```python
from build123d import *

# Parameters (mm, degrees)
F4_W      = 5.05
F4_H      = 5.35
F9_R      = 3
F10_DEPTH = 11.671
F11_R     = 0.5
F12_SIZE  = 0.2


with BuildPart() as f6:
    # F6: sweep along a path in F1
    with BuildLine(Plane.XZ) as f6_path:
        Line((0, 0), (0, 1.2))
        Line((0, 1.2), (0, 3.4))
        Line((0, 3.4), (0, 4.67))
        Line((0, 4.67), (0, 11.67))
    # F5 (on Top) → F6 (sweep)
    with BuildSketch(Plane.XY):
        Polygon((-12.95, -8.55), (0, -8.55), (12.95, -8.55), (12.95, -3.875), (18, -3.875), (18, 3.875), (12.95, 3.875), (12.95, 8.55), (-12.95, 8.55), (-12.95, 3.875), (-18, 3.875), (-18, -3.875), (-12.95, -3.875), align=None)
    sweep(path=f6_path.line)

    # F7: sweep along a path in F1
    with BuildLine(Plane.XZ) as f7_path:
        Line((0, 1.2), (0, 3.4))
        Line((0, 3.4), (0, 4.67))
        Line((0, 4.67), (0, 11.67))
    # F4 (on line) → F7 (sweep, cut)
    with BuildSketch(Plane.XY.offset(1.2)):
        Polygon((11.75, 2.675), (11.75, 7.35), (-11.75, 7.35), (-11.75, 2.675), (-11.75, -2.675), (-11.75, -7.35), (-2.65, -7.35), (-2.65, -16.2557040095), (2.65, -16.2557040095), (2.65, -7.35), (11.75, -7.35), (11.75, -2.675), align=None)
        with Locations((14.275, 0)):
            Rectangle(F4_W, F4_H)
        with Locations((-14.275, 0)):
            Rectangle(F4_W, F4_H)
    sweep(path=f7_path.line, mode=Mode.SUBTRACT)

    # F8: sweep along a path in F1
    with BuildLine(Plane.XZ) as f8_path:
        Line((0, 1.2), (0, 3.4))
    # F4 (on line) → F8 (sweep)
    with BuildSketch(Plane.XY.offset(1.2)):
        with Locations((-14.275, 0)):
            Rectangle(F4_W, F4_H)
        with Locations((14.275, 0)):
            Rectangle(F4_W, F4_H)
    sweep(path=f8_path.line)

    # F9 (on Top) → F10 (cut, through all)
    with BuildSketch(Plane.XY):
        Circle(F9_R)
    extrude(amount=F10_DEPTH, mode=Mode.SUBTRACT)

    # F11
    f11_edges = [f6.edges().sort_by_distance(p)[0] for p in [
        (-2.65, -7.35, 6.435),
        (2.65, -7.35, 6.435),
        (-11.75, 0, 3.4),
        (11.75, 0, 3.4),
        (18, -3.875, 5.835),
        (18, 3.875, 5.835),
        (12.95, -8.55, 5.835),
        (12.95, 8.55, 5.835),
        (-12.95, -8.55, 5.835),
        (-18, -3.875, 5.835),
        (-12.95, 8.55, 5.835),
        (-18, 3.875, 5.835),
        (12.95, 3.875, 5.835),
        (12.95, -3.875, 5.835),
        (-12.95, -3.875, 5.835),
        (-12.95, 3.875, 5.835),
        (11.75, 2.675, 7.535),
        (11.75, -2.675, 7.535),
        (-11.75, -2.675, 7.535),
        (-11.75, 2.675, 7.535),
    ]]
    fillet(f11_edges, radius=F11_R)

    # F12
    f12_edges = [f6.edges().sort_by_distance(p)[0] for p in [
        (0, -8.55, 0),
        (-12.803553, -8.403553, 0),
        (12.803553, -8.403553, 0),
        (-12.95, -6.2125, 0),
        (12.95, -6.2125, 0),
        (-13.096447, -4.021447, 0),
        (13.096447, -4.021447, 0),
        (-15.475, -3.875, 0),
        (15.475, -3.875, 0),
        (-17.853553, -3.728553, 0),
        (17.853553, -3.728553, 0),
        (-18, 0, 0),
        (18, 0, 0),
        (-17.853553, 3.728553, 0),
        (17.853553, 3.728553, 0),
        (-15.475, 3.875, 0),
        (15.475, 3.875, 0),
        (-13.096447, 4.021447, 0),
        (13.096447, 4.021447, 0),
        (-12.95, 6.2125, 0),
        (12.95, 6.2125, 0),
        (-12.803553, 8.403553, 0),
        (12.803553, 8.403553, 0),
        (0, 8.55, 0),
        (-3, 0, 0),
    ]]
    chamfer(f12_edges, length=F12_SIZE)


solid = f6.part
```
Geometry check sheet. Reference: the model listing, model coordinates, mm. A direction names the side the tool comes from. Give positions to 0.01 mm unless a question says otherwise; leave off trailing zeros. Loops run counter-clockwise (first coordinate to the right, second up) from the corner with the lowest first, then second, coordinate; pieces in that order, holes last. Notation, with made-up numbers: M 78,16.25 L 104,16.25 A12 ccw 104,28.25 Z; hole C 50,19 d10. An arc over 180 degrees is marked long. Answer as CSV lines item,"result".
Item 1: Cross-section at D-D on y = -6.75. Record the cut outline in (x, z), and give its area (3 significant figures).
Values:
outline,"M -12.95,0.2 L -12.75,0 L 12.75,0 L 12.95,0.2 L 12.95,11.67 L 11.75,11.67 L 11.75,1.2 L -11.75,1.2 L -11.75,11.67 L -12.95,11.67 Z"
area,"56.2 mm²"
Item 2: Cross-section at B-B on x = 0. Record the cut outline in (y, z).
Values:
outline,"M -8.55,0.2 L -8.35,0 L -3.2,0 L -3,0.2 L -3,1.2 L -8.55,1.2 Z; M 3,0.2 L 3.2,0 L 8.35,0 L 8.55,0.2 L 8.55,11.67 L 7.35,11.67 L 7.35,1.2 L 3,1.2 Z"
Item 3: Access from +Z, -Z, +X, -X, +Y, -Y to the whole of each face (thin tool, end or side, straight path). Record for faces 4 (the flat face through (-15, 3.875, 6)), 5 (the flat face through (-16, -3.875, 6)), 6 (the cylindrical face through (-3, 0, 1)), 7 (the flat face through (0, 7.35, 7)), 8 (the flat face through (15, -3.875, 6)).
Values:
face 4,"+Z, -Z, -X, +Y"
face 5,"+Z, -Z, -X, -Y"
face 6,"+Z, -Z"
face 7,"+Z"
face 8,"+Z, -Z, +X, -Y"
Item 4: Release check for a two-part mould opening along X. For faces 1 (the flat face through (-12.95, -6, 6)), 2 (the flat face through (16.8, 0, 8)), 3 (the flat face through (-3, -8.55, 6)) record: pulls with the +X half, pulls with the -X half, needs draft (parallel to the pull), parting line crosses it, or undercut.
Values:
face 1,"pulls with the -X half"
face 2,"undercut"
face 3,"needs draft"
Item 5: Depth check by flat-ended pin: P1, Ø0.6, axis at y = -8.5, z = 6, coming from the +X side; P2, Ø3.5, axis at x = 14, y = 0.5, coming from the +Z side; P3, Ø1, axis at x = 13.5, y = -5, coming from the +Z side; P4, Ø2.5, axis at x = 14, z = 6, coming from the +Y side. Enter the tip coordinate at first touch or a pass-through.
Values:
P1,"stops at x = 12.93"
P2,"stops at z = 3.4"
P3,"passes through"
P4,"stops at y = 8.45"
Item 6: Cross-section at A-A on y = 0. Record the cut outline in (x, z), and give its area (3 significant figures).
Values:
outline,"M -18,0.2 L -17.8,0 L -3.2,0 L -3,0.2 L -3,1.2 L -11.75,1.2 L -11.75,2.9 A0.5 ccw -12.25,3.4 L -16.8,3.4 L -16.8,11.67 L -18,11.67 Z; M 3,0.2 L 3.2,0 L 17.8,0 L 18,0.2 L 18,11.67 L 16.8,11.67 L 16.8,3.4 L 12.25,3.4 A0.5 ccw 11.75,2.9 L 11.75,1.2 L 3,1.2 Z"
area,"83.2 mm²"
Item 7: Cross-section at C-C on x = -7.5. Record the cut outline in (y, z), and give its area (3 significant figures).
Values:
outline,"M -8.55,0.2 L -8.35,0 L 8.35,0 L 8.55,0.2 L 8.55,11.67 L 7.35,11.67 L 7.35,1.2 L -7.35,1.2 L -7.35,11.67 L -8.55,11.67 Z"
area,"45.6 mm²"
Item 8: Material ranges on line 1 (Y direction, x = 11, z = 8.5); line 2 (Y direction, x = 15, z = 4) (3 decimals); line 3 (X direction, y = 0, z = 0.8), recorded low to high.
Values:
line 1,"y = -8.55 to -7.35, 7.35 to 8.55"
line 2,"y = -3.875 to -2.675, 2.675 to 3.875"
line 3,"x = -18 to -3, 3 to 18"
